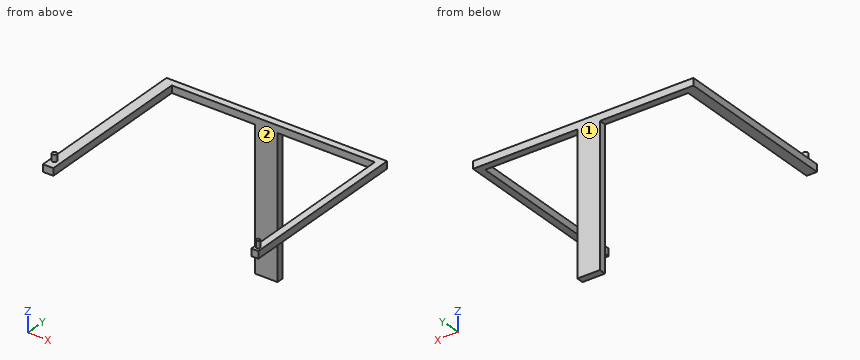
```python
from build123d import *

# Parameters (mm, degrees)
F0_W      = 37.547688
F0_H      = 26.145774
F1_DEPTH  = 609.6
F2_W      = 25.4
F2_H      = 26.145774
F3_DEPTH  = 762
F4_W      = 25.4
F4_H      = 26.145774
F5_DEPTH  = 609.6
F6_W      = 82.078397
F6_H      = 25.4
F7_DEPTH  = 508
F8_R      = 8.291485
F9_DEPTH  = 25.4
F10_R     = 6.534669
F11_DEPTH = 25.4


with BuildPart() as f1:
    # F0 (on Front) → F1 (new body)
    with BuildSketch(Plane.XZ):
        Rectangle(F0_W, F0_H)
    extrude(amount=-F1_DEPTH)

    # F2 (on face) → F3 (join)
    with BuildSketch(Plane.YZ.offset(18.773844)):
        with Locations((596.9, 0)):
            Rectangle(F2_W, F2_H)
    extrude(amount=F3_DEPTH)

    # F4 (on face) → F5 (join)
    with BuildSketch(Plane.XZ.offset(-584.2)):
        with Locations((768.073844, 0)):
            Rectangle(F4_W, F4_H)
    extrude(amount=F5_DEPTH)

    # F6 (on face) → F7 (join)
    with BuildSketch(Plane(origin=(0, 0, -13.072887), x_dir=(1, 0, 0), z_dir=(0, 0, -1))):
        with Locations((361.406744, -596.9)):
            Rectangle(F6_W, F6_H)
    extrude(amount=F7_DEPTH)

    # F8 (on face) → F9 (join)
    with BuildSketch(Plane.XY.offset(13.072887)):
        with Locations((-3.264897, 35.729956)):
            Circle(F8_R)
    extrude(amount=F9_DEPTH)

    # F10 (on face) → F11 (join)
    with BuildSketch(Plane.XY.offset(13.072887)):
        with Locations((767.283738, -8.2256)):
            Circle(F10_R)
    extrude(amount=F11_DEPTH)


solid = f1.part
```
The model under review builds one solid part; all positions refer to its coordinate system, in mm. Face numbers are marked on the shaded views. A direction names the side the tool comes from. Round coordinates to 2 decimals unless told otherwise and drop trailing zeros. Loops run counter-clockwise (first coordinate to the right, second up) from the corner with the lowest first, then second, coordinate; pieces in that order, holes last. Notation, with made-up numbers: (-38.5, 55.25) -> (-2.5, 55.25) arc R37 cw to (-2.5, 91.25) -> close; hole circle Ø2 at (-2.75, 1.25). An arc over 180 degrees is marked (long way). Answer in a Markdown table with one row per item.
1) Consider section A-A, the plane y = 544.5. Write out the cut boundary in (x, z), plus the area to 3 significant figures.
Taken from the geometry:
| item | result |
|---|---|
| outline | (-18.77, -13.07) -> (18.77, -13.07) -> (18.77, 13.07) -> (-18.77, 13.07) -> close; (755.37, -13.07) -> (780.77, -13.07) -> (780.77, 13.07) -> (755.37, 13.07) -> close |
| area | 1,650 mm² |
2) Consider section B-B, the plane x = 196. Write out the cut boundary in (y, z).
Taken from the geometry:
| item | result |
|---|---|
| outline | (584.2, -13.07) -> (609.6, -13.07) -> (609.6, 13.07) -> (584.2, 13.07) -> close |
3) Wall thickness on line 1 along Y through (x, z) = (334, -108.5): over which ranges is the line inside the solid? List them lowest first.
Taken from the geometry:
| item | result |
|---|---|
| line 1 | y = 584.2 to 609.6 |
4) For pin 1 Ø7.5 at (y, z) = (592, -163) entering from +X; pin 2 Ø21 at (x, z) = (-1, -3) entering from -Y, all flat-tipped, find the tip position at first contact; note any pin that passes through.
Taken from the geometry:
| item | result |
|---|---|
| pin 1 | stops at x = 402.45 |
| pin 2 | stops at y = 0 |
5) Tool access review of the marked faces 1 and 2: name each direction out of +Z, -Z, +X, -X, +Y, -Y from which nothing blocks a thin tool from reaching the whole face with its end or side.
Taken from the geometry:
| item | result |
|---|---|
| face 1 | +Z, -Z, +X, -X, +Y |
| face 2 | +Z, -Z, -Y |
6) Consider section C-C, the plane z = -101. Write out the cut boundary in (x, y).
Taken from the geometry:
| item | result |
|---|---|
| outline | (320.37, 584.2) -> (402.45, 584.2) -> (402.45, 609.6) -> (320.37, 609.6) -> close |
